Part model, mm, in its own coordinate system. Face numbers are marked on the shaded views. Give positions to 0.01 mm unless a question says otherwise; leave off trailing zeros. Write each loop counter-clockwise with the first axis right and the second up, starting at its lowest first coordinate (ties: lowest second). Pieces come first, ordered by that corner, then holes. Notation, with made-up numbers: M 87,31.25 L 133,31.25 A13 ccw 133,48.25 Z; hole C 6.5,41.25 d7. An arc over 180 degrees is marked long. Use CSV: the item, a comma, the result in double quotes. Start each with the question number.
1. Mould opens along Z. For the marked faces 1, 2 and 3 say: pulls with the +Z half, pulls with the -Z half, needs draft (parallel to the pull), parting line crosses it, or undercut.
2. Band-saw the part on A-A, the plane y = 0. List the corners of the cut face in (x, z).
3. Drop flat-ended pins along their axis: pin 1 Ø5 at (x, y) = (5.5, 2) entering from -Z; pin 2 Ø4 at (x, y) = (-3.5, 4) entering from -Z; pin 3 Ø2 at (y, z) = (3, 1.5) entering from +X. Give the stop position or say it passes through.
4. Band-saw the part on D-D, the plane z = -1.5. List the corners of the cut face in (x, y), then the cut area to 3 significant figures.
5. Band-saw the part on C-C, the plane z = -0.25. List the corners of the cut face in (x, y), then the cut area to 3 significant figures.
6. Drill centre lines: line 1 along Z through (x, y) = (-6.75, 6.75); line 2 along Y through (x, z) = (0, -0.8); line 3 along X through (y, z) = (-6, 2.5). Where is each one in solid material? Low to high. Write a range as from..to.
from build123d import *

# Parameters (mm, degrees)
F0_R     = 10
F0_R_2   = 9.25
F0_R_3   = 8
F1_DEPTH = 3
F2_DEPTH = 1
F3_R     = 0.5


with BuildPart() as f1:
    # F0 (on Top) → F1 (new body, symmetric)
    with BuildSketch(Plane.XY):
        Circle(F0_R)
        Circle(F0_R_2, mode=Mode.SUBTRACT)
        Circle(F0_R_2)
        Circle(F0_R_3, mode=Mode.SUBTRACT)
    extrude(amount=F1_DEPTH, both=True)

    # F0 (on Top) → F2 (cut, symmetric)
    with BuildSketch(Plane.XY):
        Circle(F0_R)
        Circle(F0_R_2, mode=Mode.SUBTRACT)
    extrude(amount=F2_DEPTH, both=True, mode=Mode.SUBTRACT)

    # F3
    f3_edges = [f1.edges().sort_by_distance(p)[0] for p in [
        (-10, 0, 3),
        (-8, 0, 3),
        (-10, 0, -3),
        (-8, 0, -3),
    ]]
    fillet(f3_edges, radius=F3_R)


solid = f1.part
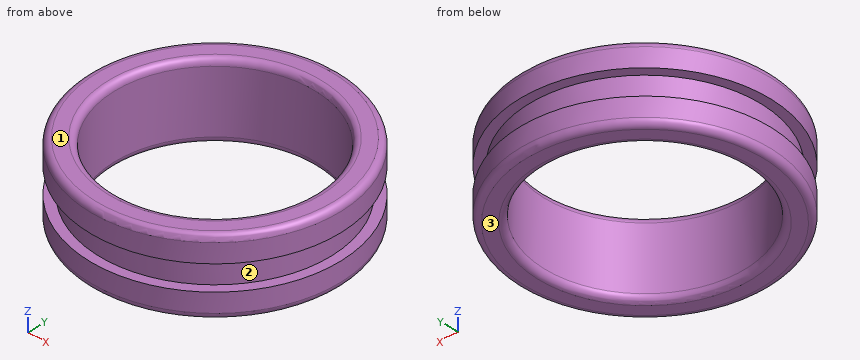
Output:
1,face 1,"pulls with the +Z half"
1,face 2,"undercut"
1,face 3,"pulls with the -Z half"
2,outline,"M -10,-2.5 A0.5 ccw -9.5,-3 L -8.5,-3 A0.5 ccw -8,-2.5 L -8,2.5 A0.5 ccw -8.5,3 L -9.5,3 A0.5 ccw -10,2.5 L -10,1 L -9.25,1 L -9.25,-1 L -10,-1 Z; M 8,-2.5 A0.5 ccw 8.5,-3 L 9.5,-3 A0.5 ccw 10,-2.5 L 10,-1 L 9.25,-1 L 9.25,1 L 10,1 L 10,2.5 A0.5 ccw 9.5,3 L 8.5,3 A0.5 ccw 8,2.5 Z"
3,pin 1,"stops at z = -2.98"
3,pin 2,"passes through"
3,pin 3,"stops at x = 9.8"
4,outline,"C 0,0 d20; hole C 0,0 d16"
4,area,"113 mm²"
5,outline,"C 0,0 d18.5; hole C 0,0 d16"
5,area,"67.7 mm²"
6,line 1,"z = -3..-1, 1..3"
6,line 2,"y = -9.25..-8, 8..9.25"
6,line 3,"x = -8..-5.29, 5.29..8"
